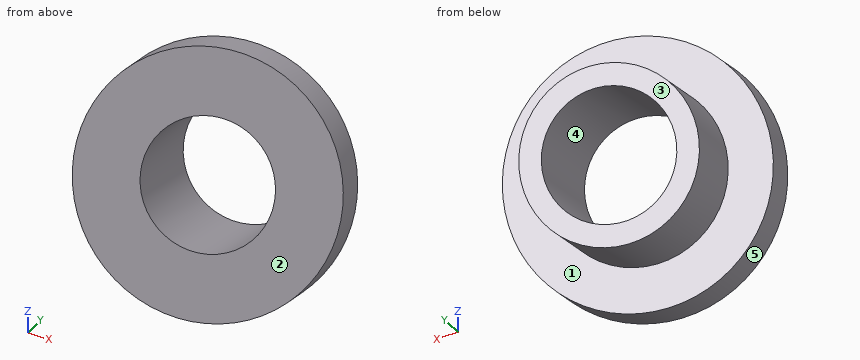
from build123d import *

# Parameters (mm, degrees)
CYLINDER026_R          = 1.5
CYLINDER026_DEPTH      = 3
CYLINDER025_R          = 2
CYLINDER025_DEPTH      = 3
CYLINDER024_R          = 3
CYLINDER024_DEPTH      = 1
CUT033_ROLL_ANGLE      = 111.214464
CUT033_PITCH_ANGLE     = 15.699901
CUT033_PLACEMENT_ANGLE = -161.024378


with BuildPart() as cylinder030:
    # Cylinder026 → Cylinder026 (new body)
    with BuildSketch(Plane.XY):
        Circle(CYLINDER026_R)
    extrude(amount=CYLINDER026_DEPTH)


with BuildPart() as cylinder029:
    # Cylinder025 → Cylinder025 (new body)
    with BuildSketch(Plane.XY):
        Circle(CYLINDER025_R)
    extrude(amount=CYLINDER025_DEPTH)


with BuildPart() as obj1:
    # Cylinder024 → Cylinder024 (new body)
    with BuildSketch(Plane.XY):
        Circle(CYLINDER024_R)
    extrude(amount=CYLINDER024_DEPTH)

    # Fusion026: union Cylinder029
    add(cylinder029.part)

    # Cut033: cut Cylinder030
    add(cylinder030.part, mode=Mode.SUBTRACT)


with BuildPart() as obj1_1:
    # Cut033 roll: moved
    add(obj1.part.rotate(Axis((0, 0, 0), (1, 0, 0)), CUT033_ROLL_ANGLE))


with BuildPart() as obj1_2:
    # Cut033 pitch: moved
    add(obj1_1.part.rotate(Axis((0, 0, 0), (0, 1, 0)), CUT033_PITCH_ANGLE))


with BuildPart() as obj1_3:
    # Cut033 placement: moved
    add(obj1_2.part.moved(Location((3e-06, -2e-06, -2.999996))).rotate(Axis((3e-06, -2e-06, -2.999996), (0, 0, 1)), CUT033_PLACEMENT_ANGLE))


solid = obj1_3.part
Read the model definition and answer for the solid it produces. Units are mm, in the model's axes. Face numbers are marked on the shaded views. A direction names the side the tool comes from. Round coordinates to 2 decimals unless told otherwise and drop trailing zeros.
1. Determine the mould class of the marked faces 3, 4 and 5 for opening direction Z: pulls with the +Z half, pulls with the -Z half, needs draft (parallel to the pull), parting line crosses it, or undercut.
2. Given pin 1 Ø1.5 at (y, z) = (1, -2) entering from -X; pin 2 Ø1 at (x, y) = (0.5, 1.5) entering from +Z, each flat-ended and moving along its own axis, determine where each tip first touches the part or whether it passes through.
3. Straight lines are drawn through the part: L1, parallel to X at y = 0.55, z = -3.8; L2, parallel to Z at x = 0, y = 2.95; L3, parallel to Y at x = 1.75, z = -4.95. For each, find the intervals that lie inside material, in ascending order.
4. Which of the six approach directions +Z, -Z, +X, -X, +Y, -Y give full straight-line access (tool end or side, diameter ignored) to the marked faces 1 and 2?
Values:
1. face 3: pulls with the -Z half
1. face 4: undercut
1. face 5: parting line crosses it
2. pin 1: stops at x = -3.09
2. pin 2: stops at z = -0.22
3. L1: x = -2.14 to -1.6, 1.25 to 2.84
3. L2: z = -2.63 to -2.06
3. L3: y = -0.34 to 0.75
4. face 1: none
4. face 2: +Z, +X, -Y
